Geometry check sheet. Reference: the model listing, model coordinates, mm. A direction names the side the tool comes from. Round coordinates to 2 decimals unless told otherwise and drop trailing zeros. Write each loop counter-clockwise with the first axis right and the second up, starting at its lowest first coordinate (ties: lowest second). Pieces come first, ordered by that corner, then holes. Notation, with made-up numbers: (-0.5, 68.25) - (58.5, 68.25) arc R30 cw to (58.5, 92.25) - close; hole circle Ø4 at (75.25, 40). An arc over 180 degrees is marked (long way). One line per question, with ' | ' between items. Start each with the question number.
Autodesk Inventor part; units mm, degrees
ref_plane "YZ Plane" through (0, 0, 0) normal (1, 0, 0) x (0, 1, 0)
ref_plane "XZ Plane" through (0, 0, 0) normal (0, 1, 0) x (-1, 0, 0)
ref_plane "XY Plane" through (0, 0, 0) normal (0, 0, 1) x (1, 0, 0)
sketch "Esboço1" plane through (0, 0, 0) normal (0, 0, 1) x (1, 0, 0)
  line L0 (0, 0) -> (-5, 0)
  line L1 (-5, 0) -> (-5, -5)
  line L2 (-5, -5) -> (-2, -5)
  line L3 (-2, -5) -> (-2, -15)
  line L4 (-2, -15) -> (-5, -15)
  line L5 (-5, -15) -> (-5, -20)
  line L6 (-5, -20) -> (0, -20)
  line L7 (0, -20) -> (0, -17)
  line L8 (0, -17) -> (10, -17)
  line L9 (10, -17) -> (10, -20)
  line L10 (10, -20) -> (15, -20)
  line L11 (15, -20) -> (15, -15)
  line L12 (15, -15) -> (12, -15)
  line L13 (12, -15) -> (12, -5)
  line L14 (12, -5) -> (15, -5)
  line L15 (15, -5) -> (15, 0)
  line L16 (15, 0) -> (10, 0)
  line L17 (10, 0) -> (10, -3)
  line L18 (10, -3) -> (0, -3)
  line L19 (0, -3) -> (0, 0)
  dimension "d4" = 5
  dimension "d5" = 5
  dimension "d6" = 3
  dimension "d7" = 10
  dimension "d8" = 3
  dimension "d9" = 5
  dimension "d10" = 5
  dimension "d11" = 3
  dimension "d12" = 10
  dimension "d13" = 5
  dimension "d14" = 5
  dimension "d15" = 3
  dimension "d16" = 10
  dimension "d17" = 3
  dimension "d18" = 5
  dimension "d19" = 3
  dimension "d20" = 10
extrude "Extrusão1" add sketch "Esboço1" along normal blind 150
sketch "Esboço5" plane through (0, 0, 150) normal (0, 0, 1) x (1, 0, 0)
  line L0 (12, -15) -> (12, -5)
  line L1 (15, -15) -> (12, -15)
  line L2 (12, -5) -> (15, -5)
  line L3 (15, -5) -> (15, -15)
  line L4 (15, -15) -> (12, -15)
  line L5 (12, -15) -> (12, -5)
  line L6 (0, -17) -> (10, -17)
  line L7 (0, -17) -> (10, -17)
  line L8 (10, -17) -> (10, -20)
  line L9 (10, -20) -> (0, -20)
  line L10 (0, -20) -> (0, -17)
  line L11 (12, -5) -> (15, -5)
  line L12 (15, -5) -> (25, -5)
  line L13 (25, -5) -> (25, -15)
  line L14 (25, -15) -> (15, -15)
  line L15 (15, -15) -> (15, -5)
  line L16 (0, -20) -> (0, -17)
  line L17 (0, -20) -> (10, -20)
  line L18 (10, -20) -> (10, -31)
  line L19 (10, -31) -> (0, -31)
  line L20 (0, -31) -> (0, -20)
  line L21 (0, -31) -> (10, -31)
  line L22 (10, -31) -> (10, -36)
  line L23 (10, -36) -> (0, -36)
  line L24 (0, -36) -> (0, -31)
  line L25 (25, -5) -> (30, -5)
  line L26 (30, -5) -> (30, -15)
  line L27 (30, -15) -> (25, -15)
  line L28 (25, -15) -> (25, -5)
  point P0 (0, 0)
extrude "Extrusão2" add sketch "Esboço5" against normal blind 15
fillet "Arredondamento1" radius 10 2 edges at (30, -10, 135) (5, -36, 135)
properties part number "viga de suporte"
Q1. Section check D-D, the plane y = -22. Record the cut outline in (x, z), then the cut area to 3 significant figures.
Q2. Section check A-A, the plane y = -1.5. Record the cut outline in (x, z), then the cut area to 3 significant figures.
Q3. Thickness scan on line 1 (X direction, y = -2, z = 120); line 2 (Y direction, x = 6, z = 118.5); line 3 (Z direction, x = 6.5, y = -26). Record the ranges inside material, lowest first.
Q4. Section check B-B, the plane x = 2.5. Record the cut outline in (y, z).
Q5. Draft check along Y on faces 4 (the flat face through (16, -10, 135)), 5 (the flat face through (-5, -2, 74)), 6 (the flat face through (13, 0, 74)), 7 (the flat face through (-4, -5, 74)). Enter one of: pulls with the +Y half, pulls with the -Y half, needs draft (parallel to the pull), parting line crosses it, or undercut.
Q6. Section check C-C, the plane z = 82. Record the cut outline in (x, y), then the cut area to 3 significant figures.
Q7. Go/stop test with flat-tipped pins: P1, Ø4, axis at y = -16.5, z = 95, coming from the +X side; P2, Ø8, axis at x = 5, z = 70, coming from the +Y side; P3, Ø1.5, axis at x = 14, z = 38, coming from the -Y side. Record where each tip stops, or that it passes through.
Q8. Set-up check for faces 1 (the flat face through (5, -21, 135)), 2 (the flat face through (10, -1, 74)), 3 (the flat face through (13, -5, 67)): record each of +Z, -Z, +X, -X, +Y, -Y from which the full face is reachable in a straight line by a thin tool's end or side.
Result sheet:
1) outline: (0, 135) - (10, 135) - (10, 150) - (0, 150) - close | area: 150 mm²
2) outline: (-5, 0) - (0, 0) - (0, 150) - (-5, 150) - close; (10, 0) - (15, 0) - (15, 150) - (10, 150) - close | area: 1,500 mm²
3) line 1: -5 to 0, 10 to 15 | line 2: -17 to -3 | line 3: 135 to 150
4) outline: (-36, 145) arc R10 ccw to (-26, 135) - (-17, 135) - (-17, 0) - (-3, 0) - (-3, 150) - (-36, 150) - close
5) face 4: undercut | face 5: needs draft | face 6: pulls with the +Y half | face 7: undercut
6) outline: (-5, -20) - (0, -20) - (0, -17) - (10, -17) - (10, -20) - (15, -20) - (15, -15) - (12, -15) - (12, -5) - (15, -5) - (15, 0) - (10, 0) - (10, -3) - (0, -3) - (0, 0) - (-5, 0) - (-5, -5) - (-2, -5) - (-2, -15) - (-5, -15) - close | area: 280 mm²
7) P1: x = 15 | P2: y = -3 | P3: y = -20
8) face 1: -Z, -Y | face 2: +Z, -Z, +Y | face 3: -Z, +X
